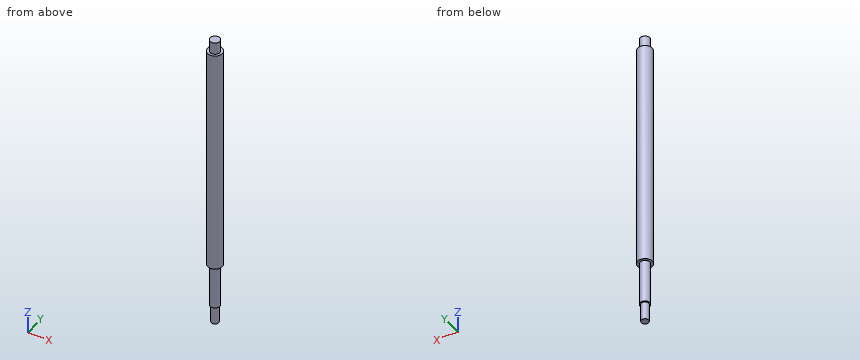
from build123d import *

# Parameters (mm, degrees)
SKETCH1_R           = 6
BOSS_EXTRUDE1_DEPTH = 250
SKETCH2_OUTSIDE_W   = 64.116
SKETCH2_OUTSIDE_H   = 64.116
SKETCH2_OUTSIDE_R   = 3
F_6MM_DEPTH         = 15
SKETCH3_OUTSIDE_W   = 64.116
SKETCH3_OUTSIDE_H   = 64.116
SKETCH3_OUTSIDE_R   = 4
F_8MM_DEPTH         = 51
SKETCH4_OUTSIDE_W   = 64.116
SKETCH4_OUTSIDE_H   = 64.116
SKETCH4_OUTSIDE_R   = 4
F_8MM_IDLE_DEPTH    = 10


with BuildPart() as part:
    # Sketch1 → Boss-Extrude1 (new body)
    with BuildSketch(Plane.XY):
        Circle(SKETCH1_R)
    extrude(amount=BOSS_EXTRUDE1_DEPTH)

    # Sketch2 outside → 6mm (cut)
    with BuildSketch(Plane(origin=(0, 0, 0), x_dir=(-1, 0, 0), z_dir=(0, 0, -1))):
        Rectangle(SKETCH2_OUTSIDE_W, SKETCH2_OUTSIDE_H)
        Circle(SKETCH2_OUTSIDE_R, mode=Mode.SUBTRACT)
    extrude(amount=-F_6MM_DEPTH, mode=Mode.SUBTRACT)

    # Sketch3 outside → 8mm (cut)
    with BuildSketch(Plane(origin=(0, 0, 0), x_dir=(-1, 0, 0), z_dir=(0, 0, -1))):
        Rectangle(SKETCH3_OUTSIDE_W, SKETCH3_OUTSIDE_H)
        Circle(SKETCH3_OUTSIDE_R, mode=Mode.SUBTRACT)
    extrude(amount=-F_8MM_DEPTH, mode=Mode.SUBTRACT)

    # Sketch4 outside → 8mm-Idle (cut)
    with BuildSketch(Plane.XY.offset(250)):
        Rectangle(SKETCH4_OUTSIDE_W, SKETCH4_OUTSIDE_H)
        with Locations(Location((0, 0, 0), (0, 0, 180))):
            Circle(SKETCH4_OUTSIDE_R, mode=Mode.SUBTRACT)
    extrude(amount=-F_8MM_IDLE_DEPTH, mode=Mode.SUBTRACT)


solid = part.part
Design review of the part built by this model. Coordinates are the model's own, in mm. Give positions to 0.01 mm unless a question says otherwise; leave off trailing zeros. Loops run counter-clockwise (first coordinate to the right, second up) from the corner with the lowest first, then second, coordinate; pieces in that order, holes last. Notation, with made-up numbers: M -9.5,-30.5 L 17.5,-30.5 A14 cw 17.5,-5.5 Z; hole C -23,-39 d9. An arc over 180 degrees is marked long. Write item = value, one per line.
Q1. We need section D-D (z = 209). Give the boundary of the cut face in (x, y), plus the area to 3 significant figures.
Output values:
outline = C 0,0 d12
area = 113 mm^2
Q2. We need section C-C (z = 45.5). Give the boundary of the cut face in (x, y), plus the area to 3 significant figures.
Output values:
outline = C 0,0 d8
area = 50.3 mm^2
Q3. Insertion check: pin 1 (4 mm diameter, centred on x = -4.5, z = 160, fed in from +Y); pin 2 (6 mm diameter, centred on x = -3, z = 90, fed in from -Y); pin 3 (4 mm diameter, centred on y = 4, z = 195, fed in from -X); pin 4 (1 mm diameter, centred on y = 2.5, z = 96.5, fed in from +X). Each pin has a flat end and moves straight along its axis. Give the tip position at first contact, or say it passes through.
Output values:
pin_1 = 5.45
pin_2 = -6
pin_3 = -5.66
pin_4 = 5.66
Q4. To check wall thickness, follow line 1 (Y direction, x = 0.5, z = 100); line 2 (Z direction, x = 3, y = -5). State the ranges of each line that lie inside material, in increasing order. Write a range as [from, to].
Output values:
line_1 = [-5.98, 5.98]
line_2 = [51, 240]
Q5. We need section A-A (x = 0). Give the boundary of the cut face in (y, z), plus the area to 3 significant figures.
Output values:
outline = M -6,51 L -4,51 L -4,15 L -3,15 L -3,0 L 3,0 L 3,15 L 4,15 L 4,51 L 6,51 L 6,240 L 4,240 L 4,250 L -4,250 L -4,240 L -6,240 Z
area = 2,730 mm^2
